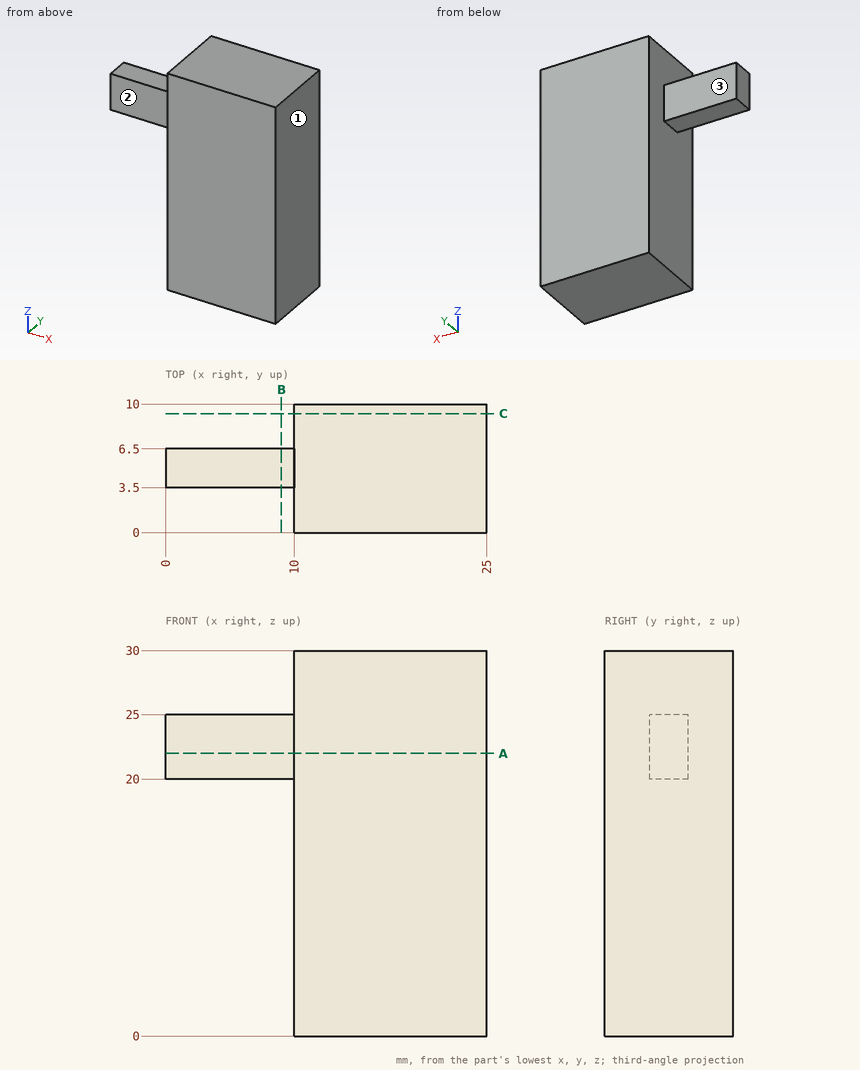
Print and shaded views of the part. All mm, measured from the part's lowest x, y and z. A direction names the side the tool comes from. Coordinates: 2 decimals unless noted, no trailing zeros. Loops run counter-clockwise (first coordinate to the right, second up) from the corner with the lowest first, then second, coordinate; pieces in that order, holes last. Notation, with made-up numbers: (18.25, 65) -> (64.25, 65) arc R29 ccw to (64.25, 86) -> close; hole circle Ø8 at (58, 25). An arc over 180 degrees is marked (long way). Use one line per item in the form item = value. Start each with the question number.
(1) Probe probe 1 along X at (y, z) = (2.5, 27.5); probe 2 along Y at (x, z) = (8.75, 22); probe 3 along Z at (x, y) = (5.75, 5.5). List the from-to ranges inside material, lowest first. Write a range as from..to.
(2) Cut at C-C on y = 9.25. Give the cut face in (x, z).
(3) Cut at A-A on z = 22. Give the cut face in (x, y), and give its area (3 significant figures).
(4) Flat gauge pins, fed straight in: pin 1 (1 mm diameter, centred on y = 5.5, z = 27, fed in from -X); pin 2 (0.9 mm diameter, centred on x = 4.5, y = 5.5, fed in from -Z); pin 3 (4 mm diameter, centred on x = 6.5, z = 23.5, fed in from +Y). Where does each tip first touch, or does it go through?
(5) Tool access for the marked faces 1, 2 and 3: list every direction of +Z, -Z, +X, -X, +Y, -Y with a clear straight run to the whole face (end or side of a thin tool).
(6) Cut at B-B on x = 9. Give the cut face in (y, z).
Values:
q1.probe_1 = 10..25
q1.probe_2 = 3.5..6.5
q1.probe_3 = 20..25
q2.outline = (10, 0) -> (25, 0) -> (25, 30) -> (10, 30) -> close
q3.outline = (0, 3.5) -> (10, 3.5) -> (10, 0) -> (25, 0) -> (25, 10) -> (10, 10) -> (10, 6.5) -> (0, 6.5) -> close
q3.area = 180 mm2
q4.pin_1 = 10
q4.pin_2 = 20
q4.pin_3 = 6.5
q5.face_1 = +Z, -Z, +X, +Y, -Y
q5.face_2 = +Z, -Z, -X, -Y
q5.face_3 = +Z, -Z, -X, +Y
q6.outline = (3.5, 20) -> (6.5, 20) -> (6.5, 25) -> (3.5, 25) -> close
